Here's how the part is built. I have some questions about the finished solid (model axes, mm). Face numbers are marked on the shaded views. A direction names the side the tool comes from. Coordinates: 2 decimals unless noted, no trailing zeros. Write each loop counter-clockwise with the first axis right and the second up, starting at its lowest first coordinate (ties: lowest second). Pieces come first, ordered by that corner, then holes. Notation, with made-up numbers: M -27.75,33 L 12.25,33 A20 ccw 12.25,67 Z; hole C 19.25,-34 d11. An arc over 180 degrees is marked long. Use one line per item in the form item = value. Start each with the question number.
1. I'm going to push a flat-ended pin straight in: pin 1 Ø8.5 at (x, y) = (-76, 67) entering from +Z. Where does the tip first touch, or does it pass through?
2. I want a section at D-D, the plane x = -70.5. List the corners of the cut face in (y, z) for me, plus the area to 3 significant figures.
3. On a 3-axis mill with a long thin cutter (end or side, diameter ignored), from which of +Z, -Z, +X, -X, +Y, -Y can I reach the whole of each face in a straight line? I mean the marked faces 4 and 5. Say none if no direction works.
4. Please list where these lines run through material, in increasing order: line 1 along X through (y, z) = (78, 47); line 2 along Y through (x, z) = (-66.5, 41); line 3 along Y through (x, z) = (-67.75, 55). Write a range as [from, to].
5. I want a section at C-C, the plane x = -64. List the corners of the cut face in (y, z) for me.
6. I want a section at A-A, the plane z = 4. List the corners of the cut face in (x, y) for me, plus the area to 3 significant figures.
7. I want a section at B-B, the plane y = 74. List the corners of the cut face in (x, z) for me, plus the area to 3 significant figures.
8. Thinking about a two-plate mould opening in X: for the marked faces 1, 2 and 3, which applies, released by +X, released by -X, zero draft, split by the parting line, or undercut?
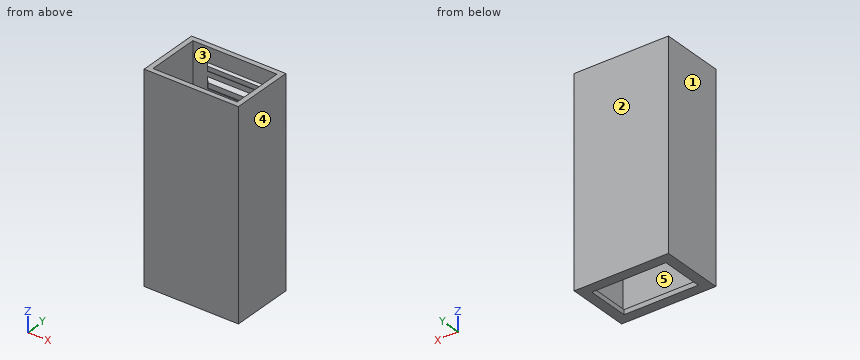
from build123d import *

# Parameters (mm, degrees)
F0_W         = 30
F0_H         = 20
F1_DEPTH     = 65
F0_W_2       = 23.6
F0_H_2       = 13.6
F0_W_3       = 16.8
F0_H_3       = 1
F2_DEPTH     = 1.5
F4_W         = 0.6
F4_H         = 3
F4_W_2       = 1
F4_H_2       = 4
F5_DEPTH     = 9
F6_T4_DEPTH  = 22.1146927807
F6_T9_DEPTH  = 22.1146927807
F6_T14_DEPTH = 7.1146927807
F6_T19_DEPTH = 7.1146927807
F7_T4_DEPTH  = 24.1720391711
F7_T9_DEPTH  = 24.1720391711
F7_T14_DEPTH = 10.1720391711
F7_T19_DEPTH = 10.1720391711


# Not quite as in the source:
# - a fillet or chamfer that OpenCascade refuses, or shapes differently, is made with other operations: its cross-section is extruded or revolved along the edge and cut away or added


with BuildPart() as f1:
    # F0 (on Top) → F1 (new body)
    with BuildSketch(Plane.XY):
        with Locations((-75, 70)):
            Rectangle(F0_W, F0_H)
        Polygon((-88.4, 61.6), (-88.4, 78.4), (-83.4, 78.4), (-66.6, 78.4), (-61.6, 78.4), (-61.6, 61.6), align=None, mode=Mode.SUBTRACT)
    extrude(amount=F1_DEPTH)

    # F0 (on Top) → F2 (join)
    with BuildSketch(Plane.XY):
        Polygon((-83.4, 78.4), (-88.4, 78.4), (-88.4, 61.6), (-61.6, 61.6), (-61.6, 78.4), (-66.6, 78.4), (-66.6, 77.4), (-83.4, 77.4), align=None)
        with Locations((-75, 70)):
            Rectangle(F0_W_2, F0_H_2, mode=Mode.SUBTRACT)
        with Locations((-75, 77.9)):
            Rectangle(F0_W_3, F0_H_3)
    extrude(amount=F2_DEPTH)

    # F4 (on mid) → F5 (join, symmetric)
    with BuildSketch(Plane.YZ.offset(-75)):
        with Locations((78.1, 58.9)):
            Rectangle(F4_W, F4_H)
        with Locations((77.9, 54.2)):
            Rectangle(F4_W_2, F4_H_2)
    extrude(amount=F5_DEPTH, both=True)

    # F6: chamfer of 0.8 on 4 edges, made by hand


with BuildPart() as f6_tool2:
    # F6_s3 → F6_t4 (new body)
    with BuildSketch(Plane.YZ.offset(-86.0573463904)):
        Polygon((78.6, 60.4), (77.8, 59.6), (77.8, 60.4), align=None)
    extrude(amount=F6_T4_DEPTH)

    split(bisect_by=Plane.XZ.offset(-78.4), keep=Keep.TOP)


with BuildPart() as f1_1:
    add(f1.part)

    # F6_t1: cut F6_tool2
    add(f6_tool2.part, mode=Mode.SUBTRACT)


with BuildPart() as f6_tool7:
    # F6_s8 → F6_t9 (new body)
    with BuildSketch(Plane.YZ.offset(-63.9426536096)):
        Polygon((78.6, 57.4), (77.8, 58.2), (77.8, 57.4), align=None)
    extrude(amount=-F6_T9_DEPTH)

    split(bisect_by=Plane.XZ.offset(-78.4), keep=Keep.TOP)


with BuildPart() as f1_2:
    add(f1_1.part)

    # F6_t6: cut F6_tool7
    add(f6_tool7.part, mode=Mode.SUBTRACT)


with BuildPart() as f6_tool12:
    # F6_s13 → F6_t14 (new body)
    with BuildSketch(Plane.XY.offset(62.4573463904)):
        Polygon((-84, 78.6), (-83.2, 77.8), (-84, 77.8), align=None)
    extrude(amount=-F6_T14_DEPTH)

    split(bisect_by=Plane.XZ.offset(-78.4), keep=Keep.TOP)


with BuildPart() as f1_3:
    add(f1_2.part)

    # F6_t11: cut F6_tool12
    add(f6_tool12.part, mode=Mode.SUBTRACT)


with BuildPart() as f6_tool17:
    # F6_s18 → F6_t19 (new body)
    with BuildSketch(Plane.XY.offset(62.4573463904)):
        Polygon((-66, 78.6), (-66.8, 77.8), (-66, 77.8), align=None)
    extrude(amount=-F6_T19_DEPTH)

    split(bisect_by=Plane.XZ.offset(-78.4), keep=Keep.TOP)


with BuildPart() as f1_4:
    add(f1_3.part)

    # F6_t16: cut F6_tool17
    add(f6_tool17.part, mode=Mode.SUBTRACT)

    # F7: chamfer of 1.2 on 4 edges, made by hand


with BuildPart() as f7_tool2:
    # F7_s3 → F7_t4 (new body)
    with BuildSketch(Plane.YZ.offset(-87.0860195856)):
        Polygon((78.6, 56.2), (77.4, 55), (77.4, 56.2), align=None)
    extrude(amount=F7_T4_DEPTH)

    split(bisect_by=Plane.XZ.offset(-78.4), keep=Keep.TOP)


with BuildPart() as f1_5:
    add(f1_4.part)

    # F7_t1: cut F7_tool2
    add(f7_tool2.part, mode=Mode.SUBTRACT)


with BuildPart() as f7_tool7:
    # F7_s8 → F7_t9 (new body)
    with BuildSketch(Plane.YZ.offset(-62.9139804144)):
        Polygon((78.6, 52.2), (77.4, 53.4), (77.4, 52.2), align=None)
    extrude(amount=-F7_T9_DEPTH)

    split(bisect_by=Plane.XZ.offset(-78.4), keep=Keep.TOP)


with BuildPart() as f1_6:
    add(f1_5.part)

    # F7_t6: cut F7_tool7
    add(f7_tool7.part, mode=Mode.SUBTRACT)


with BuildPart() as f7_tool12:
    # F7_s13 → F7_t14 (new body)
    with BuildSketch(Plane.XY.offset(59.2860195856)):
        Polygon((-84, 78.6), (-82.8, 77.4), (-84, 77.4), align=None)
    extrude(amount=-F7_T14_DEPTH)

    split(bisect_by=Plane.XZ.offset(-78.4), keep=Keep.TOP)


with BuildPart() as f1_7:
    add(f1_6.part)

    # F7_t11: cut F7_tool12
    add(f7_tool12.part, mode=Mode.SUBTRACT)


with BuildPart() as f7_tool17:
    # F7_s18 → F7_t19 (new body)
    with BuildSketch(Plane.XY.offset(59.2860195856)):
        Polygon((-66, 78.6), (-67.2, 77.4), (-66, 77.4), align=None)
    extrude(amount=-F7_T19_DEPTH)

    split(bisect_by=Plane.XZ.offset(-78.4), keep=Keep.TOP)


with BuildPart() as f1_8:
    add(f1_7.part)

    # F7_t16: cut F7_tool17
    add(f7_tool17.part, mode=Mode.SUBTRACT)


solid = f1_8.part
Answer list:
q1.pin_1 = 1.5
q2.outline = M 60,0 L 63.2,0 L 63.2,1.5 L 61.6,1.5 L 61.6,65 L 60,65 Z; M 76.8,0 L 80,0 L 80,65 L 78.4,65 L 78.4,60.2 L 77.8,59.6 L 77.8,58.2 L 78.4,57.6 L 78.4,56 L 77.4,55 L 77.4,53.4 L 78.4,52.4 L 78.4,1.5 L 76.8,1.5 Z
q2.area = 217 mm²
q3.face_4 = +Z, -Z, +X, +Y, -Y
q3.face_5 = +Z
q4.line_1 = [-90, -88.4], [-61.6, -60]
q4.line_2 = [60, 61.6], [78.4, 80]
q4.line_3 = [60, 61.6], [77.4, 80]
q5.outline = M 60,0 L 63.2,0 L 63.2,1.5 L 61.6,1.5 L 61.6,65 L 60,65 Z; M 76.8,0 L 80,0 L 80,65 L 78.4,65 L 78.4,1.5 L 76.8,1.5 Z
q6.outline = M -90,60 L -60,60 L -60,80 L -90,80 Z; hole M -88.4,61.6 L -61.6,61.6 L -61.6,78.4 L -88.4,78.4 Z
q6.area = 150 mm²
q7.outline = M -90,0 L -86.8,0 L -86.8,1.5 L -88.4,1.5 L -88.4,65 L -90,65 Z; M -63.2,0 L -60,0 L -60,65 L -61.6,65 L -61.6,1.5 L -63.2,1.5 Z
q7.area = 213 mm²
q8.face_1 = released by -X
q8.face_2 = zero draft
q8.face_3 = undercut
